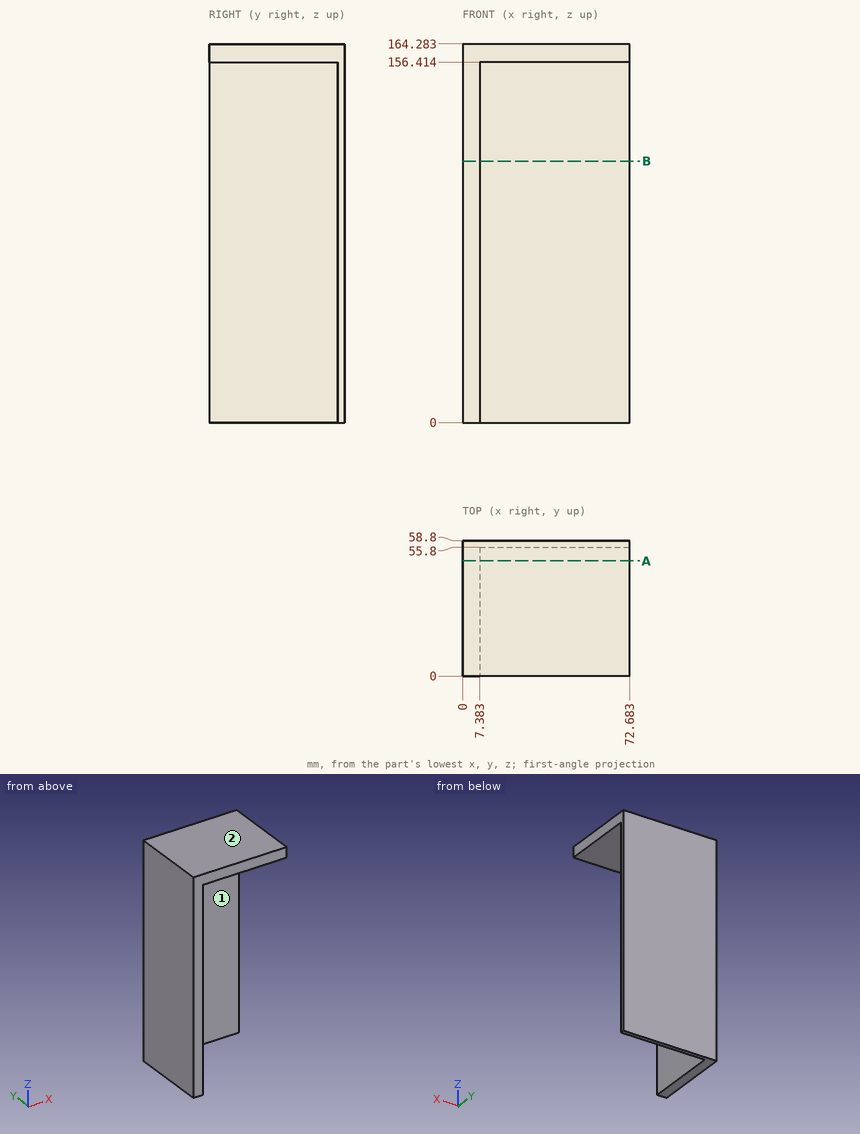
Input: dimensioned drawing with shaded views. Units: mm. Origin: part minimum x, y, z. A direction names the side the tool comes from. Coordinates: 2 decimals unless noted, no trailing zeros. Order: outer loops, then holes, each group sorted by start corner. A loop starts at its lowest first (then second) coordinate and runs counter-clockwise, first axis right, second up. Notation, with made-up numbers: M 31,-35.75 L 75,-35.75 A16 cw 75,-10.75 Z; hole C 82,36 d1. An arc over 180 degrees is marked long. Write each question's results on one line, items separated by ' | '. Start each with the question number.
Item 1: Cut plane A-A (y = 50). Return loops of the section in (x, z).
Item 2: Line query: probe 1 along X at (y, z) = (17, 43.5); probe 2 along Y at (x, z) = (42, 63); probe 3 along Z at (x, y) = (54, 43.5). Output: solid intervals per line, ascending.
Item 3: First-contact query: pin 1 Ø2 at (x, z) = (40.5, 132.5) entering from -Y; pin 2 Ø2 at (x, y) = (43, 31.5) entering from -Z; pin 3 Ø2 at (y, z) = (12, 30) entering from -X. Flat tips, straight axial feed; report the tip coordinate or a pass-through.
Item 4: Cut plane B-B (z = 113.5). Return loops of the section in (x, y).
Item 5: Set-up query: the marked faces 1 and 2. Return all of +Z, -Z, +X, -X, +Y, -Y with unobstructed straight access to the full face (end or side cutting, diameter ignored); none if empty.
Checked values:
1) outline: M 0,0 L 7.38,0 L 7.38,156.41 L 72.68,156.41 L 72.68,164.28 L 0,164.28 Z
2) probe 1: x = 0 to 7.38 | probe 2: y = 55.8 to 58.8 | probe 3: z = 156.41 to 164.28
3) pin 1: stops at y = 55.8 | pin 2: stops at z = 156.41 | pin 3: stops at x = 0
4) outline: M 0,0 L 7.38,0 L 7.38,55.8 L 72.68,55.8 L 72.68,58.8 L 0,58.8 Z
5) face 1: -Z, +X, -Y | face 2: +Z, +X, -X, +Y, -Y
